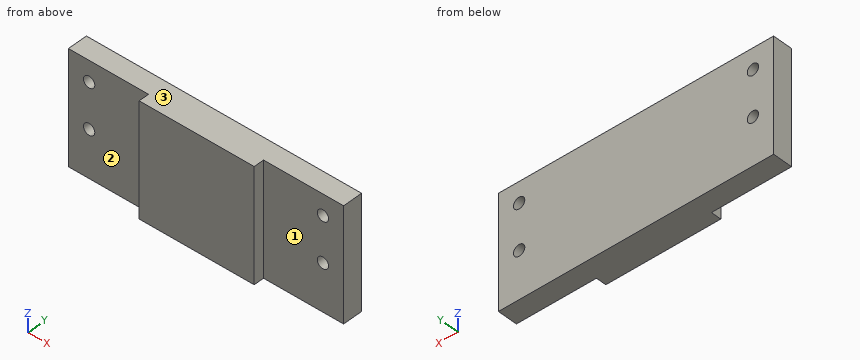
from build123d import *

# Parameters (mm, degrees)
SKETCH_1_W          = 73
SKETCH_1_H          = 30
EXTRUDE_1_DEPTH     = 8
SKETCH_2_W          = 21.25
SKETCH_2_H          = 2.735303139
CUT_EXTRUDE_1_DEPTH = 48.919202831
SKETCH_3_R          = 1.5
CUT_EXTRUDE_2_DEPTH = 45


with BuildPart() as part:
    # 草图1 → 凸台-拉伸1 (new body)
    with BuildSketch(Plane(origin=(0, 0, 0), x_dir=(1, 0, 0), z_dir=(0, 1, 0))):
        Rectangle(SKETCH_1_W, SKETCH_1_H)
    extrude(amount=EXTRUDE_1_DEPTH)

    # 草图2 → 切除-拉伸1 (cut, through all)
    with BuildSketch(Plane(origin=(0, 0, -15), x_dir=(-1, 0, 0), z_dir=(0, 0, -1))):
        with Locations((-25.875, 1.367651569)):
            Rectangle(SKETCH_2_W, SKETCH_2_H)
        with Locations((25.875, 1.367651569)):
            Rectangle(SKETCH_2_W, SKETCH_2_H)
    extrude(amount=-CUT_EXTRUDE_1_DEPTH, mode=Mode.SUBTRACT)

    # 草图3 → 切除-拉伸2 (cut, symmetric)
    with BuildSketch(Plane(origin=(59.282070169, -20, -16.5), x_dir=(1, 0, 0), z_dir=(0, -1, 0))):
        with Locations((-28.282070169, 14)):
            Circle(SKETCH_3_R)
        with Locations((-90.282070169, 14)):
            Circle(SKETCH_3_R)
        with Locations((-90.282070169, 26)):
            Circle(SKETCH_3_R)
        with Locations((-28.282070169, 26)):
            Circle(SKETCH_3_R)
    extrude(amount=CUT_EXTRUDE_2_DEPTH, both=True, mode=Mode.SUBTRACT)


solid = part.part
Geometry: final body of the model. Coordinates: model frame, mm. Face numbers are marked on the shaded views. A direction names the side the tool comes from. Round coordinates to 2 decimals unless told otherwise and drop trailing zeros. Order: outer loops, then holes, each group sorted by start corner. A loop starts at its lowest first (then second) coordinate and runs counter-clockwise, first axis right, second up. Notation, with made-up numbers: (-11.75, 5) -> (-5.75, 5) arc R35 ccw to (-5.75, 37) -> close; hole circle Ø7 at (65.5, -0.75). An arc over 180 degrees is marked (long way). Put each result on its own line as item: value. Start each with the question number.
Q1. Section A-A on x = -31. Return the cut outline in (y, z).
Q2. Reachability of the marked faces 1, 2 and 3 from +Z, -Z, +X, -X, +Y, -Y: full face, straight path, thin tool, end or side. Return the list, or none.
Q3. First-contact query: pin 1 (3.5 mm diameter, centred on x = -31, z = -2.5, fed in from -Y); pin 2 (0.8 mm diameter, centred on y = 1.5, z = -1, fed in from -X); pin 3 (0.8 mm diameter, centred on y = 1, z = -2, fed in from +X). Flat tips, straight axial feed; report the tip coordinate or a pass-through.
Q4. Section C-C on z = -8.5. Return the cut outline in (x, y), and give its area (3 significant figures).
Q5. Line query: probe 1 along Z at (x, y) = (31, 5.6); probe 2 along X at (y, z) = (7.25, 8.5); probe 3 along Y at (x, z) = (25.5, -6.75). Output: solid intervals per line, ascending.
Q6. Section B-B on z = 9.5. Return the cut outline in (x, y).
Q7. Section D-D on y = 1.25. Return the cut outline in (x, z), and give its area (3 significant figures).
Ans:
1. outline: (2.74, -15) -> (8, -15) -> (8, -4) -> (2.74, -4) -> close; (2.74, -1) -> (8, -1) -> (8, 8) -> (2.74, 8) -> close; (2.74, 11) -> (8, 11) -> (8, 15) -> (2.74, 15) -> close
2. face 1: +Z, -Z, +X, -Y
2. face 2: +Z, -Z, -X, -Y
2. face 3: +Z, +X, -X, +Y, -Y
3. pin 1: stops at y = 2.74
3. pin 2: stops at x = -15.25
3. pin 3: stops at x = 15.25
4. outline: (-36.5, 2.74) -> (-15.25, 2.74) -> (-15.25, 0) -> (15.25, 0) -> (15.25, 2.74) -> (36.5, 2.74) -> (36.5, 8) -> (-36.5, 8) -> close
4. area: 468 mm2
5. probe 1: z = -15 to -4, -1 to 8, 11 to 15
5. probe 2: x = -36.5 to -32.12, -29.88 to 29.88, 32.12 to 36.5
5. probe 3: y = 2.74 to 8
6. outline: (-36.5, 2.74) -> (-32.5, 2.74) -> (-32.5, 8) -> (-36.5, 8) -> close; (-29.5, 2.74) -> (-15.25, 2.74) -> (-15.25, 0) -> (15.25, 0) -> (15.25, 2.74) -> (29.5, 2.74) -> (29.5, 8) -> (-29.5, 8) -> close; (32.5, 2.74) -> (36.5, 2.74) -> (36.5, 8) -> (32.5, 8) -> close
7. outline: (-15.25, -15) -> (15.25, -15) -> (15.25, 15) -> (-15.25, 15) -> close
7. area: 915 mm2
